CAD build for the part. Positions are in the model's coordinates, mm. A direction names the side the tool comes from. Coordinates: 2 decimals unless noted, no trailing zeros. Answer as a JSON object with one key per item and string values. Group by question number.
from build123d import *


with BuildPart() as f1:
    # F0 (on Front) → F1 (revolve)
    with BuildSketch(Plane.XZ):
        with BuildLine():
            add(Edge.make_bspline(
                [(-22.9642885055, 49.3032115787), (-12.2969623123, 46.4702763814), (-22.4618348296, 0), (-18.1075624479, 0)],
                knots=[2.9191818186, 2.9191818186, 2.9191818186, 2.9191818186, 49.811763635, 49.811763635, 49.811763635, 49.811763635], degree=3))
            Line((-18.1075624479, 0), (-58.0540070499, 0))
            add(Edge.make_bspline(
                [(-58.0540070499, 0), (-77.442342212, -11.0468430516), (-61.7601881483, -58.9445413015), (-14.4063218335, 1.1245636718), (-2.5255118479, -22.637057851)],
                knots=[0, 0, 0, 0, 0.4307775151, 1, 1, 1, 1], degree=3))
            Line((-2.5255118479, -22.637057851), (-1.5875, -34.4977003213))
            Line((-1.5875, -34.4977003213), (-1.5875, -17.4797003213))
            Line((-1.5875, -17.4797003213), (0, -17.4797003213))
            Line((0, -17.4797003213), (0, 35.7623191787))
            Line((0, 35.7623191787), (-4.73075, 35.7623191787))
            Line((-4.73075, 35.7623191787), (-4.73075, 49.3032115787))
            add(Edge.make_bspline(
                [(-4.73075, 49.3032115787), (-10.7331998616, 49.3032115787), (-17.0701686457, 49.3032115787), (-22.9642885055, 49.3032115787)],
                knots=[4.8317135305, 4.8317135305, 4.8317135305, 4.8317135305, 22.8923422862, 22.8923422862, 22.8923422862, 22.8923422862], degree=3))
        make_face()
    revolve(axis=Axis((0, 0, 9.1413094287), (0, 0, -1)))


solid = f1.part
Item 1: Drill centre lines: L1, parallel to Y at x = 0, z = -25.75; L2, parallel to Y at x = 0, z = 44.25; L3, parallel to Y at x = 0, z = -21. Where is each one in solid material? Low to high.
Item 2: 3-axis set-ups, long thin cutter, end or side, ignore diameter. For faces 1 (the flat face through (0, 0, 35.762)), 2 (the conical face through (-1.89, -0.79, -28.65)): which of +Z, -Z, +X, -X, +Y, -Y reach the whole face in a straight line?
Item 3: Pull direction X, two halves, no side cores. Call faces 3 (the cylindrical face through (-4.512, 1.421, 42.628)), 4 (the flat face through (-14, 14, 0)): +X half, -X half, draft (parallel to the pull), parting line (faces both ways), or undercut.
Item 4: Band-saw the part on A-A, the plane y = 19. Count the separate pieces of the cut face and the enclosed holes in it, and give its area (3 significant figures).
Item 5: Flat gauge pins, fed straight in: P1, Ø4, axis at x = -41, y = 32, coming from the -Z side; P2, Ø1, axis at x = 0.5, y = -0.5, coming from the -Z side; P3, Ø3, axis at x = -23, y = -41.5, coming from the +Z side; P4, Ø4, axis at x = 23, y = 6.5, coming from the +Z side. Where does each tip first touch, or does it go through?
Reply:
{
 "1": {"L1": "-68.18 to -40.42, -2.28 to -1.59, 1.59 to 2.28, 40.42 to 68.18", "L2": "-19.08 to -4.73, 4.73 to 19.08", "L3": "-69.91 to -32.36, -3.42 to -1.59, 1.59 to 3.42, 32.36 to 69.91"},
 "2": {"face 1": "+Z", "face 2": "-Z"},
 "3": {"face 3": "undercut", "face 4": "draft"},
 "4": {"separate pieces": "3", "enclosed holes": "0", "area": "3,190 mm²"},
 "5": {"P1": "z = -31.88", "P2": "z = -17.48", "P3": "z = 0", "P4": "z = 49.3"}
}
